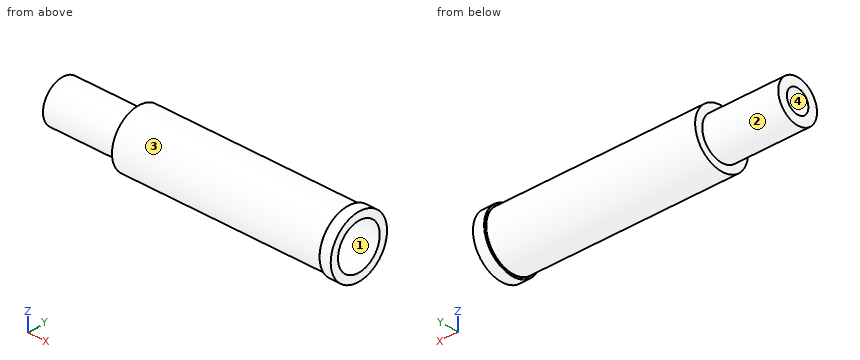
```python
from build123d import *

# Parameters (mm, degrees)
F2_W = 100
F2_H = 6.1
F5_R = 0.2


# Not quite as in the source:
# - a feature of the source that left no trace in its solid (it failed there, or was rolled back) is left out


with BuildPart() as f1:
    # F0 (on Top) → F1 (revolve)
    with BuildSketch(Plane.XY):
        Polygon((53, -16), (53, 0), (47, 0), (0, 0), (-103, 0), (-103, -11), (-63, -11), (-63, -15), (47, -15), (47, -16), align=None)
    revolve(axis=Axis((-51.5, 0, 0), (-1, 0, 0)))

    # F2 (on Front) → F3 (revolve, cut)
    with BuildSketch(Plane.XZ):
        Polygon((53, 11.85), (-34, 9.6771213406), (-34, 6.1), (-34, 0), (0, 0), (53, 0), align=None)
        with Locations((-84, 3.05)):
            Rectangle(F2_W, F2_H)
    revolve(axis=Axis((26.5, 0, 0), (-1, 0, 0)), mode=Mode.SUBTRACT)

    # F5
    f5_edges = [f1.edges().sort_by_distance(p)[0] for p in [
        (47, 16, 0),
        (47, 15, 0),
    ]]
    fillet(f5_edges, radius=F5_R)


solid = f1.part
```
Geometry check sheet. Reference: the model listing, model coordinates, mm. Face numbers are marked on the shaded views. A direction names the side the tool comes from. Round coordinates to 2 decimals unless told otherwise and drop trailing zeros. Order: outer loops, then holes, each group sorted by start corner. A loop starts at its lowest first (then second) coordinate and runs counter-clockwise, first axis right, second up. Notation, with made-up numbers: (5.25, -15) -> (21.25, -15) arc R23 ccw to (21.25, 3) -> close; hole circle Ø4 at (57, -9.75). An arc over 180 degrees is marked (long way). Return JSON: item names as keys, results as strings. Group by question number.
Q1. Section check A-A, the plane y = 0. Record the boundary of the cut face in (x, z), plus the area to 3 significant figures.
Q2. Section check D-D, the plane x = 21.5. Record the boundary of the cut face in (y, z).
Q3. Gauge pin test, flat ends, axial feed: pin 1 (5 mm diameter, centred on x = 3, z = -9, fed in from +Y); pin 2 (5 mm diameter, centred on x = -66, z = -4, fed in from +Y); pin 3 (10 mm diameter, centred on x = 21, z = -7, fed in from -Y); pin 4 (2 mm diameter, centred on y = -5, z = 10, fed in from -X). Record the tip position at first contact, or that the pin passes through.
Q4. Material ranges on probe 1 along Z at (x, y) = (-75, 0); probe 2 along X at (y, z) = (12.5, -7); probe 3 along Z at (x, y) = (10.5, -7), recorded low to high. Write a range as from..to.
Q5. Tool access check on the marked faces 1 and 2. Record the directions out of +Z, -Z, +X, -X, +Y, -Y that give a thin tool (end or side, any length) a straight path to the whole face; none if there is none.
Q6. Release check for a two-part mould opening along Y. For the marked faces 3 and 4 record: released by +Y, released by -Y, zero draft, split by the parting line, or undercut.
Q7. Section check C-C, the plane x = -48.5. Record the boundary of the cut face in (y, z), plus the area to 3 significant figures.
Numbers:
{
 "1": {"outline": "(-103, -11) -> (-63, -11) -> (-63, -15) -> (46.8, -15) arc R0.2 cw to (47, -15.2) -> (47, -15.8) arc R0.2 ccw to (47.2, -16) -> (53, -16) -> (53, -11.85) -> (-34, -9.68) -> (-34, -6.1) -> (-103, -6.1) -> close; (-103, 6.1) -> (-34, 6.1) -> (-34, 9.68) -> (53, 11.85) -> (53, 16) -> (47.2, 16) arc R0.2 ccw to (47, 15.8) -> (47, 15.2) arc R0.2 cw to (46.8, 15) -> (-63, 15) -> (-63, 11) -> (-103, 11) -> close", "area": "1,660 mm^2"},
 "2": {"outline": "circle Ø30 at (0, 0); hole circle Ø22.13 at (0, 0)"},
 "3": {"pin 1": "y = 13.52", "pin 2": "y = 10.9", "pin 3": "y = -14.87", "pin 4": "x = -103"},
 "4": {"probe 1": "-11..-6.1, 6.1..11", "probe 2": "-63..53", "probe 3": "-13.27..-8.21, 8.21..13.27"},
 "5": {"face 1": "+X", "face 2": "-X"},
 "6": {"face 3": "split by the parting line", "face 4": "undercut"},
 "7": {"outline": "circle Ø30 at (0, 0); hole circle Ø12.2 at (0, 0)", "area": "590 mm^2"}
}
